from build123d import *
from build123d.topology import SkipClean

# Parameters (mm, degrees)
SKETCH_1_R               = 40.9
SKETCH_1_R_2             = 1.525
EXTRUDE_1_DEPTH          = 1.5
EXTRUDE_START            = -1.5
EXTRUDE_2_DEPTH          = 1.5
CUT_EXTRUDE_1_DEPTH      = 70.399279535
CUT_EXTRUDE_1_DEPTH_BACK = 70.399279535
SKETCH_3_R               = 1.525
SKETCH_4_R               = 40.9
SKETCH_4_R_2             = 1.525
EXTRUDE_3_DEPTH          = 10.5
CUT_EXTRUDE_START        = -12
CUT_EXTRUDE_2_DEPTH      = 12
EXTRUDE_4_DEPTH          = 2.5
EXTRUDE_5_REACH          = 106.449
EXTRUDE_5_END_RADIUS     = 48
SKETCH_8_R               = 1
CUT_EXTRUDE_3_DEPTH      = 105.448711512
CHAMFER_1_SIZE           = 1.2
CHAMFER_1_SIZE_2         = 2.827022839
CHAMFER_2_SIZE           = 1.091910703
CHAMFER_2_SIZE_2         = 3
SKETCH_9_W               = 24
SKETCH_9_H               = 12
EXTRUDE_6_DEPTH          = 17.5
SKETCH_10_R              = 1.55
CUT_EXTRUDE_4_DEPTH      = 90.170454762
SKETCH_11_W              = 17.5
SKETCH_11_H              = 12
SKETCH_11_R              = 1.55
EXTRUDE_7_DEPTH          = 3.9
EXTRUDE_START_2          = 3.4
SKETCH_12_W              = 17.5
SKETCH_12_H              = 12
SKETCH_12_R              = 1.55
EXTRUDE_8_DEPTH          = 3.4
FILLET_1_R               = 2


with BuildPart() as part:
    # 草图1 → 凸台-拉伸1 (new body)
    with BuildSketch(Plane(origin=(0, 0, 0), x_dir=(1, 0, 0), z_dir=(0, 1, 0))):
        with BuildLine():
            Line((12, 50.1), (-12, 50.1))
            ThreePointArc((-12, 50.1), (-12.071709603, 48.790080839), (-12.285981368, 47.495817309))
            ThreePointArc((-12.285981368, 47.495817309), (-12.775478285, 46.565992731), (-13.668785094, 46.012653847))
            ThreePointArc((-13.668785094, 46.012653847), (0.147817484, -47.999772395), (13.385132402, 46.095967617))
            ThreePointArc((13.385132402, 46.095967617), (12.311228539, 46.859989672), (11.945854344, 48.126283833))
            ThreePointArc((11.945854344, 48.126283833), (11.98646104, 49.112770637), (12, 50.1))
        make_face()
        with Locations(Location((0, 0, 0), (0, 0, 270))):
            Circle(SKETCH_1_R, mode=Mode.SUBTRACT)
        with Locations(Location((12.835117837, 41.981778787, 0), (0, 0, 270))):
            Circle(SKETCH_1_R_2, mode=Mode.SUBTRACT)
        with Locations(Location((-17.153096541, 40.410163067, 0), (0, 0, 270))):
            Circle(SKETCH_1_R_2, mode=Mode.SUBTRACT)
    extrude(amount=EXTRUDE_1_DEPTH)

    # 草图2 → 凸台-拉伸2 (add)
    with BuildSketch(Plane(origin=(0, 1.5, 0), x_dir=(1, 0, 0), z_dir=(0, 1, 0)).offset(EXTRUDE_START)):
        with BuildLine():
            Line((-19.201386918, 36.112556548), (-17.121235913, 32.200361501))
            ThreePointArc((-17.121235913, 32.200361501), (-16.264760822, 31.479428059), (-15.147630365, 31.55232629))
            ThreePointArc((-15.147630365, 31.55232629), (-0.252986109, 34.999085674), (14.689928016, 31.768003004))
            ThreePointArc((14.689928016, 31.768003004), (15.348239226, 31.629764257), (16.000770136, 31.793125857))
            Line((16.000770136, 31.793125857), (21.673697907, 34.685167133))
            ThreePointArc((21.673697907, 34.685167133), (1.427389415, 40.875084825), (-19.201386918, 36.112556548))
        make_face()
    extrude(amount=EXTRUDE_2_DEPTH)

    # 草图3 → 切除-拉伸1 (cut, two sides: drawn at the far end of the back side and taken through both)
    with BuildSketch(Plane(origin=(0, 1.5, 0), x_dir=(1, 0, 0), z_dir=(0, 1, 0)).offset(-CUT_EXTRUDE_1_DEPTH_BACK)):
        with Locations(Location((31.749094475, 31.749094475, 0), (0, 0, 270))):
            Circle(SKETCH_3_R)
        with Locations(Location((31.749094475, -31.749094475, 0), (0, 0, 270))):
            Circle(SKETCH_3_R)
        with Locations(Location((-31.749094475, -31.749094475, 0), (0, 0, 270))):
            Circle(SKETCH_3_R)
        with Locations(Location((-31.749094475, 31.749094475, 0), (0, 0, 270))):
            Circle(SKETCH_3_R)
    extrude(amount=CUT_EXTRUDE_1_DEPTH + CUT_EXTRUDE_1_DEPTH_BACK, mode=Mode.SUBTRACT)

    # 草图4 → 凸台-拉伸3 (add)
    with SkipClean():  # the faces are left unmerged after this step: merging them gives an invalid solid
        with BuildSketch(Plane(origin=(0, 1.5, 0), x_dir=(1, 0, 0), z_dir=(0, 1, 0))):
            with BuildLine():
                Line((12, 50.1), (-12, 50.1))
                ThreePointArc((-12, 50.1), (-12.071709603, 48.790080839), (-12.285981368, 47.495817309))
                ThreePointArc((-12.285981368, 47.495817309), (-12.775478285, 46.565992731), (-13.668785094, 46.012653847))
                ThreePointArc((-13.668785094, 46.012653847), (0.147817484, -47.999772395), (13.385132402, 46.095967617))
                ThreePointArc((13.385132402, 46.095967617), (12.311228539, 46.859989672), (11.945854344, 48.126283833))
                ThreePointArc((11.945854344, 48.126283833), (11.98646104, 49.112770637), (12, 50.1))
            make_face()
            with Locations(Location((0, 0, 0), (0, 0, 118))):
                Circle(SKETCH_4_R, mode=Mode.SUBTRACT)
            with Locations(Location((-17.153096541, 40.410163067, 0), (0, 0, 270))):
                Circle(SKETCH_4_R_2, mode=Mode.SUBTRACT)
            with Locations(Location((12.835117837, 41.981778787, 0), (0, 0, 270))):
                Circle(SKETCH_4_R_2, mode=Mode.SUBTRACT)
            with Locations(Location((31.749094475, 31.749094475, 0), (0, 0, 270))):
                Circle(SKETCH_4_R_2, mode=Mode.SUBTRACT)
            with Locations(Location((31.749094475, -31.749094475, 0), (0, 0, 270))):
                Circle(SKETCH_4_R_2, mode=Mode.SUBTRACT)
            with Locations(Location((-31.749094475, -31.749094475, 0), (0, 0, 270))):
                Circle(SKETCH_4_R_2, mode=Mode.SUBTRACT)
            with Locations(Location((-31.749094475, 31.749094475, 0), (0, 0, 270))):
                Circle(SKETCH_4_R_2, mode=Mode.SUBTRACT)
        extrude(amount=EXTRUDE_3_DEPTH)
    add(part.part.scale(1), mode=Mode.REPLACE)  # the faces are merged on a copy

    # 草图5 → 切除-拉伸2 (cut)
    with BuildSketch(Plane(origin=(0, 12, 0), x_dir=(1, 0, 0), z_dir=(0, 1, 0)).offset(CUT_EXTRUDE_START)):
        with BuildLine():
            ThreePointArc((-33.864147525, 29.482698526), (-34.848632515, 31.695578705), (-33.941125497, 33.941125497))
            ThreePointArc((-33.941125497, 33.941125497), (-48, 0), (-33.941125497, -33.941125497))
            ThreePointArc((-33.941125497, -33.941125497), (-34.848632515, -31.695578705), (-33.864147525, -29.482698526))
            ThreePointArc((-33.864147525, -29.482698526), (-44.9, 0), (-33.864147525, 29.482698526))
        make_face()
        with BuildLine():
            ThreePointArc((33.864147525, -29.482698526), (34.848632515, -31.695578705), (33.941125497, -33.941125497))
            ThreePointArc((33.941125497, -33.941125497), (48, 0), (33.941125497, 33.941125497))
            ThreePointArc((33.941125497, 33.941125497), (34.848632515, 31.695578705), (33.864147525, 29.482698526))
            ThreePointArc((33.864147525, 29.482698526), (44.9, 0), (33.864147525, -29.482698526))
        make_face()
        with BuildLine():
            ThreePointArc((-29.482698526, -33.864147525), (-31.695578705, -34.848632515), (-33.941125497, -33.941125497))
            ThreePointArc((-33.941125497, -33.941125497), (0, -48), (33.941125497, -33.941125497))
            ThreePointArc((33.941125497, -33.941125497), (31.695578705, -34.848632515), (29.482698526, -33.864147525))
            ThreePointArc((29.482698526, -33.864147525), (0, -44.9), (-29.482698526, -33.864147525))
        make_face()
    extrude(amount=CUT_EXTRUDE_2_DEPTH, mode=Mode.SUBTRACT)

    # 草图6 → 凸台-拉伸4 (add)
    with BuildSketch(Plane.XZ):
        with BuildLine():
            Line((-20, -35.676462829), (-24.203821377, -32.969456027))
            ThreePointArc((-24.203821377, -32.969456027), (-22.14331564, -34.387258868), (-20, -35.676462829))
        make_face()
    extrude(amount=-EXTRUDE_4_DEPTH)

    # 凸台-拉伸5: up to this cylinder (the profile starts inside it)
    extrude_5_end = Plane(origin=(0, -1.061033, 0), z_dir=(0, -1, 0)) * Cylinder(EXTRUDE_5_END_RADIUS, 309.898, mode=Mode.PRIVATE)
    # 草图7 → 凸台-拉伸5 (add, up to the surface)
    with BuildSketch(Plane(origin=(-22.101910689, 0, -34.322959428), x_dir=(0.8407642754995167, 0, -0.5414013604007409), z_dir=(0.5414013604007408, 0, 0.8407642754995166)), mode=Mode.PRIVATE) as extrude_5_sk1:
        with BuildLine():
            Line((-2.5, 0), (2.5, 0))
            ThreePointArc((2.5, 0), (0, -2.5), (-2.5, 0))
        make_face()
    extrude_5_tool1 = extrude(extrude_5_sk1.sketch, amount=-EXTRUDE_5_REACH, mode=Mode.PRIVATE) & extrude_5_end
    add(extrude_5_tool1.solids().sort_by_distance((-22.101911, -1.061033, -34.322959))[0])

    # 草图8 → 切除-拉伸3 (cut, through all)
    with BuildSketch(Plane(origin=(-22.101910689, 0, -34.322959428), x_dir=(0.8407642754995167, 0, -0.5414013604007409), z_dir=(0.5414013604007408, 0, 0.8407642754995166))):
        Circle(SKETCH_8_R)
    extrude(amount=-CUT_EXTRUDE_3_DEPTH, mode=Mode.SUBTRACT)

    # 倒角1
    # the kernel refuses this chamfer: 2.827022839, 1.2 mm, written as the material it takes off along each edge
    with BuildSketch(Plane(origin=(0, 1.5, 0), x_dir=(-0.6107443245214345, 0, -0.7918278664361699), z_dir=(-0.7918278664361699, 0, 0.6107443245214345))) as chamfer_1_piece_1:
        Polygon((35, CHAMFER_1_SIZE), (35 + CHAMFER_1_SIZE_2, 0), (35, 0), align=None)
    revolve(axis=Axis((0, 1.5, 0), (0, -1, 0)), revolution_arc=74.458388902, mode=Mode.SUBTRACT)

    # 倒角2
    # the kernel refuses this chamfer: 3, 1.091910703 mm, written as the material it adds along each edge
    with BuildSketch(Plane(origin=(0, 1.5, 0), x_dir=(0.6807767680816117, 0, -0.7324909501422905), z_dir=(0.7324909501422905, 0, 0.6807767680816117))) as chamfer_2_piece_1_section:
        Polygon((40.9, CHAMFER_2_SIZE), (40.9 - CHAMFER_2_SIZE_2, 0), (40.9, 0), align=None)
    chamfer_2_piece_1 = revolve(axis=Axis((0, 1.5, 0), (0, 1, 0)), revolution_arc=70.9043723, mode=Mode.PRIVATE)
    chamfer_2_piece_1 = split(chamfer_2_piece_1, bisect_by=Plane(origin=(7.492047447, 2.005552707, -27.455404982), z_dir=(-0.45418251766199275, 0, -0.8909086601050715)), keep=Keep.TOP, mode=Mode.PRIVATE)
    add(chamfer_2_piece_1)

    # 草图9 → 凸台-拉伸6 (add)
    with BuildSketch(Plane(origin=(0, 0, -50.1), x_dir=(-1, 0, 0), z_dir=(0, 0, -1))):
        with Locations((0, 6)):
            Rectangle(SKETCH_9_W, SKETCH_9_H)
    extrude(amount=EXTRUDE_6_DEPTH)

    # 草图10 → 切除-拉伸4 (cut, through all)
    with BuildSketch(Plane(origin=(12, 0, 0), x_dir=(0, 0, -1), z_dir=(1, 0, 0))):
        with Locations((56.5, 5)):
            Circle(SKETCH_10_R)
    extrude(amount=-CUT_EXTRUDE_4_DEPTH, mode=Mode.SUBTRACT)

    # 草图11 → 凸台-拉伸7 (add)
    with SkipClean():  # the faces are left unmerged after this step: merging them gives an invalid solid
        with BuildSketch(Plane.ZY.offset(12)):
            with Locations((-58.85, 6)):
                Rectangle(SKETCH_11_W, SKETCH_11_H)
            with Locations(Location((-56.5, 5, 0), (0, 0, 180))):
                Circle(SKETCH_11_R, mode=Mode.SUBTRACT)
        extrude(amount=EXTRUDE_7_DEPTH)

    # 草图12 → 凸台-拉伸8 (add)
    with SkipClean():  # the faces are left unmerged after this step: merging them gives an invalid solid
        with BuildSketch(Plane(origin=(12, 0, 0), x_dir=(0, 0, -1), z_dir=(1, 0, 0)).offset(EXTRUDE_START_2)):
            with Locations((58.85, 6)):
                Rectangle(SKETCH_12_W, SKETCH_12_H)
            with Locations((56.5, 5)):
                Circle(SKETCH_12_R, mode=Mode.SUBTRACT)
        extrude(amount=-EXTRUDE_8_DEPTH)

    # 圆角1
    fillet_1_edges = [part.edges().sort_by_distance(p)[0] for p in [
        (-15.9, 6, -67.6),
        (15.4, 6, -67.6),
    ]]
    fillet(fillet_1_edges, radius=FILLET_1_R)


solid = part.part
The listing builds one solid part. Answer for the finished solid, in the listing's coordinates (mm). A direction names the side the tool comes from. Give positions to 0.01 mm unless a question says otherwise; leave off trailing zeros. Loops run counter-clockwise (first coordinate to the right, second up) from the corner with the lowest first, then second, coordinate; pieces in that order, holes last. Notation, with made-up numbers: (-39.5, 53) - (-34.5, 53) arc R22 ccw to (-34.5, 71) - close; hole circle Ø3 at (-22, 79.25). An arc over 180 degrees is marked (long way). Use one line per item in the form item = value.
1. Given pin 1 Ø2 at (x, y) = (-15, 7) entering from +Z; pin 2 Ø3 at (y, z) = (5.5, 4) entering from +X; pin 3 Ø3 at (y, z) = (5, -56.5) entering from -X; pin 4 Ø5 at (y, z) = (9, -19) entering from +X, each flat-ended and moving along its own axis, determine where each tip first touches the part or whether it passes through.
Calculated:
pin_1 = 42.66
pin_2 = 44.83
pin_3 = through
pin_4 = 41.76
2. The mould has two halves that part along X. Classify faces 4 (the face through (24.58, 5.92, -41.23)), 5 (the face through (1.606, 1.553, -38.012)), 6 (the face through (-24, -2.5, -37.3)): pulls with the +X half, pulls with the -X half, needs draft (parallel to the pull), parting line crosses it, or undercut.
Calculated:
face_4 = pulls with the +X half
face_5 = undercut
face_6 = parting line crosses it
3. Find the intervals of material crossed by line 1 along Y through (x, z) = (-23, -36); line 2 along Z through (x, y) = (0, 4); line 3 along Y through (x, z) = (-13.6, -56.5), in increasing order. Write a range as [from, to].
Calculated:
line_1 = [-2.5, -0.99], [0.99, 12]
line_2 = [-67.6, -57.68], [-55.32, -40.9], [40.9, 44.9]
line_3 = [0, 3.45], [6.55, 12]
4. Which of the six approach directions +Z, -Z, +X, -X, +Y, -Y give full straight-line access (tool end or side, diameter ignored) to faces 1 (the face through (0.111, 0.375, -35.177)), 2 (the face through (-15.9, 6, -58)), 3 (the face through (-14, 6, -50.1))?
Calculated:
face_1 = +Y
face_2 = -Z, -X, +Y, -Y
face_3 = -X, +Y, -Y
5. Section A-A on x = 0 is taken. Give the vertices of the cut face in (y, z), then the cut area to 3 significant figures.
Calculated:
outline = (0, -67.6) - (12, -67.6) - (12, -40.9) - (2.59, -40.9) - (1.5, -37.9) - (1.5, -37.83) - (0.3, -35) - (0, -35) - close; (0, 40.9) - (12, 40.9) - (12, 44.9) - (0, 44.9) - close; hole circle Ø3.1 at (5, -56.5)
area = 370 mm^2
6. Section B-B on z = -56.5 is taken. Give the vertices of the cut face in (x, y).
Calculated:
outline = (-15.9, 0) - (15.4, 0) - (15.4, 3.45) - (-15.9, 3.45) - close; (-15.9, 6.55) - (15.4, 6.55) - (15.4, 12) - (-15.9, 12) - close
7. Section D-D on z = 0 is taken. Give the vertices of the cut face in (x, y).
Calculated:
outline = (-44.9, 0) - (-40.9, 0) - (-40.9, 12) - (-44.9, 12) - close; (40.9, 0) - (44.9, 0) - (44.9, 12) - (40.9, 12) - close
8. Section C-C on y = 5 is taken. Count the separate pieces of the cut face and the enclosed holes in it, then the cut area to 3 significant figures.
Calculated:
separate_pieces = 2
enclosed_holes = 7
area = 1,820 mm^2
